Source: CAD feature listing. Evaluate the final solid. Frame: model axes, mm. Face numbers are marked on the shaded views. A direction names the side the tool comes from. Round coordinates to 2 decimals unless told otherwise and drop trailing zeros. Loops run counter-clockwise (first coordinate to the right, second up) from the corner with the lowest first, then second, coordinate; pieces in that order, holes last.
(1) Set-up query: the marked faces 1 and 2. Return all of +Z, -Z, +X, -X, +Y, -Y with unobstructed straight access to the full face (end or side cutting, diameter ignored); none if empty.
(2) Material intervals for probe 1 along Y at (x, z) = (60, 9); probe 2 along Y at (x, z) = (-60, 5.25); probe 3 along Y at (x, z) = (-50, 8.05), sorted ascending.
(3) First-contact query: pin 1 Ø8 at (x, y) = (-50, 0) entering from -Z; pin 2 Ø4.5 at (x, y) = (60, -25) entering from -Z; pin 3 Ø1.5 at (x, z) = (61, 7) entering from -Y. Flat tips, straight axial feed; report the tip coordinate or a pass-through.
(4) Section A-A, the plane x = -50. Return the cut outline in (y, z), plus the area to 3 significant figures.
(5) Mould query, pull axis X, two halves, no side actions, for the marked faces 3, 4, 5 and 6. Classes: pulls with the +X half, pulls with the -X half, needs draft (parallel to the pull), parting line crosses it, or undercut.
(6) Section C-C, the plane z = 8. Count the separate pieces of the cut face and the enclosed holes in it, plus the area to 3 significant figures.
(7) Section B-B, the plane y = 25. Return the cut outline in (x, z).
(8) Section D-D, the plane z = 17. Return the cut outline in (x, y), plus the area to 3 significant figures.
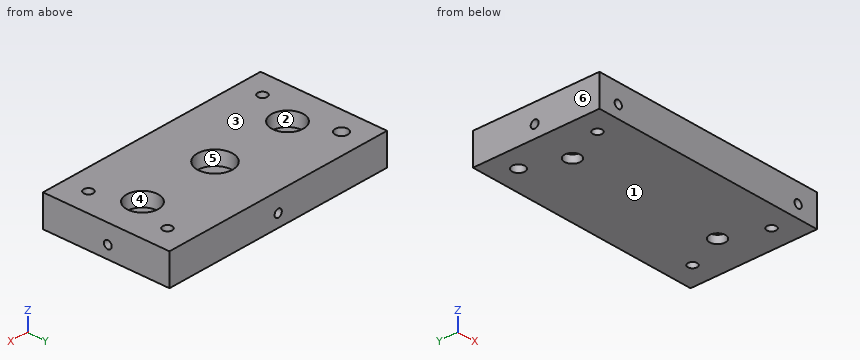
```python
from build123d import *

# Parameters (mm, degrees)
SKETCH1_W           = 150
SKETCH1_H           = 80
BOSS_EXTRUDE1_DEPTH = 20
CUT_EXTRUDE1_REACH  = 89.321
SKETCH2_R           = 3
SKETCH3_R           = 11.1
SKETCH3_R_2         = 10
CUT_EXTRUDE2_DEPTH  = 9
CUT_EXTRUDE3_REACH  = 89.321
SKETCH4_R           = 4
SKETCH4_R_2         = 2.949605035
SKETCH5_R           = 5
CUT_EXTRUDE4_DEPTH  = 5
SKETCH6_R           = 2.5
CUT_EXTRUDE5_DEPTH  = 10
SKETCH7_R           = 2.5
CUT_EXTRUDE6_DEPTH  = 10
SKETCH8_R           = 2.5
CUT_EXTRUDE7_DEPTH  = 10


with BuildPart() as part:
    # Sketch1 → Boss-Extrude1 (new body)
    with BuildSketch(Plane.XY):
        Rectangle(SKETCH1_W, SKETCH1_H)
    extrude(amount=BOSS_EXTRUDE1_DEPTH)

    # Sketch2 → Cut-Extrude1 (cut, up to next)
    with BuildSketch(Plane.XY.offset(20), mode=Mode.PRIVATE) as cut_extrude1_sk1:
        with Locations((-50, 0)):
            Circle(SKETCH2_R)
    cut_extrude1_tool1 = extrude(cut_extrude1_sk1.sketch, amount=-CUT_EXTRUDE1_REACH, mode=Mode.PRIVATE) & part.part
    # Sketch2 → Cut-Extrude1 (cut, up to next)
    with BuildSketch(Plane.XY.offset(20), mode=Mode.PRIVATE) as cut_extrude1_sk2:
        with Locations((50, 0)):
            Circle(SKETCH2_R)
    cut_extrude1_tool2 = extrude(cut_extrude1_sk2.sketch, amount=-CUT_EXTRUDE1_REACH, mode=Mode.PRIVATE) & part.part
    add(cut_extrude1_tool1.solids().sort_by_distance((-50, 0, 20))[0], mode=Mode.SUBTRACT)
    add(cut_extrude1_tool2.solids().sort_by_distance((50, 0, 20))[0], mode=Mode.SUBTRACT)

    # Sketch3 → Cut-Extrude2 (cut)
    with BuildSketch(Plane.XY.offset(20)):
        Circle(SKETCH3_R)
        with Locations((-50, 0)):
            Circle(SKETCH3_R_2)
        with Locations((50, 0)):
            Circle(SKETCH3_R_2)
    extrude(amount=-CUT_EXTRUDE2_DEPTH, mode=Mode.SUBTRACT)

    # Sketch4 → Cut-Extrude3 (cut, up to next)
    with BuildSketch(Plane.XY.offset(20), mode=Mode.PRIVATE) as cut_extrude3_sk1:
        with Locations((-60, 25)):
            Circle(SKETCH4_R)
    cut_extrude3_tool1 = extrude(cut_extrude3_sk1.sketch, amount=-CUT_EXTRUDE3_REACH, mode=Mode.PRIVATE) & part.part
    # Sketch4 → Cut-Extrude3 (cut, up to next)
    with BuildSketch(Plane.XY.offset(20), mode=Mode.PRIVATE) as cut_extrude3_sk2:
        with Locations((60, 25)):
            Circle(SKETCH4_R_2)
    cut_extrude3_tool2 = extrude(cut_extrude3_sk2.sketch, amount=-CUT_EXTRUDE3_REACH, mode=Mode.PRIVATE) & part.part
    # Sketch4 → Cut-Extrude3 (cut, up to next)
    with BuildSketch(Plane.XY.offset(20), mode=Mode.PRIVATE) as cut_extrude3_sk3:
        with Locations((60, -25)):
            Circle(SKETCH4_R_2)
    cut_extrude3_tool3 = extrude(cut_extrude3_sk3.sketch, amount=-CUT_EXTRUDE3_REACH, mode=Mode.PRIVATE) & part.part
    # Sketch4 → Cut-Extrude3 (cut, up to next)
    with BuildSketch(Plane.XY.offset(20), mode=Mode.PRIVATE) as cut_extrude3_sk4:
        with Locations((-60, -25)):
            Circle(SKETCH4_R_2)
    cut_extrude3_tool4 = extrude(cut_extrude3_sk4.sketch, amount=-CUT_EXTRUDE3_REACH, mode=Mode.PRIVATE) & part.part
    add(cut_extrude3_tool1.solids().sort_by_distance((-60, 25, 20))[0], mode=Mode.SUBTRACT)
    add(cut_extrude3_tool2.solids().sort_by_distance((60, 25, 20))[0], mode=Mode.SUBTRACT)
    add(cut_extrude3_tool3.solids().sort_by_distance((60, -25, 20))[0], mode=Mode.SUBTRACT)
    add(cut_extrude3_tool4.solids().sort_by_distance((-60, -25, 20))[0], mode=Mode.SUBTRACT)

    # Sketch5 → Cut-Extrude4 (cut)
    with BuildSketch(Plane(origin=(0, 0, 0), x_dir=(-1, 0, 0), z_dir=(0, 0, -1))):
        with Locations((-50, 0)):
            Circle(SKETCH5_R)
        with Locations((50, 0)):
            Circle(SKETCH5_R)
    extrude(amount=-CUT_EXTRUDE4_DEPTH, mode=Mode.SUBTRACT)

    # Sketch6 → Cut-Extrude5 (cut)
    with BuildSketch(Plane.ZY.offset(75)):
        with Locations((8, 1)):
            Circle(SKETCH6_R)
    cut_extrude5 = extrude(amount=-CUT_EXTRUDE5_DEPTH, mode=Mode.SUBTRACT)

    # Mirror1: Cut-Extrude5 across plane
    add(cut_extrude5.mirror(Plane(origin=(0, 0, 0), x_dir=(0, 0, 1), z_dir=(1, 0, 0))), mode=Mode.SUBTRACT)

    # Sketch7 → Cut-Extrude6 (cut)
    with BuildSketch(Plane.XZ.offset(40)):
        with Locations((-62, 8)):
            Circle(SKETCH7_R)
        with Locations(Location((62, 8, 0), (0, 0, 180))):
            Circle(SKETCH7_R)
    extrude(amount=-CUT_EXTRUDE6_DEPTH, mode=Mode.SUBTRACT)

    # Sketch8 → Cut-Extrude7 (cut)
    with BuildSketch(Plane(origin=(0, 40, 0), x_dir=(1, 0, 0), z_dir=(0, 1, 0))):
        with Locations(Location((0, -8, 0), (0, 0, 180))):
            Circle(SKETCH8_R)
    extrude(amount=-CUT_EXTRUDE7_DEPTH, mode=Mode.SUBTRACT)


solid = part.part
```
Output values:
1. face 1: -Z, +X, -X, +Y, -Y
1. face 2: +Z
2. probe 1: y = -30 to -27.95, -22.05 to 22.05, 27.95 to 40
2. probe 2: y = -40 to -27.95, -22.05 to 21, 29 to 40
2. probe 3: y = -40 to -3, 3 to 40
3. pin 1: stops at z = 5
3. pin 2: passes through
3. pin 3: stops at y = -30
4. outline: (-40, 0) - (-5, 0) - (-5, 5) - (-3, 5) - (-3, 11) - (-10, 11) - (-10, 20) - (-40, 20) - close; (3, 5) - (5, 5) - (5, 0) - (40, 0) - (40, 20) - (10, 20) - (10, 11) - (3, 11) - close
4. area: 1,330 mm2
5. face 3: needs draft
5. face 4: undercut
5. face 5: undercut
5. face 6: pulls with the -X half
6. separate pieces: 1
6. enclosed holes: 6
6. area: 11,600 mm2
7. outline: (-75, 0) - (-64, 0) - (-64, 20) - (-75, 20) - close; (-56, 0) - (57.05, 0) - (57.05, 20) - (-56, 20) - close; (62.95, 0) - (75, 0) - (75, 20) - (62.95, 20) - close
8. outline: (-75, -40) - (75, -40) - (75, 40) - (-75, 40) - close; hole circle Ø8 at (-60, 25); hole circle Ø5.9 at (-60, -25); hole circle Ø20 at (-50, 0); hole circle Ø22.2 at (0, 0); hole circle Ø20 at (50, 0); hole circle Ø5.9 at (60, -25); hole circle Ø5.9 at (60, 25)
8. area: 10,900 mm2
